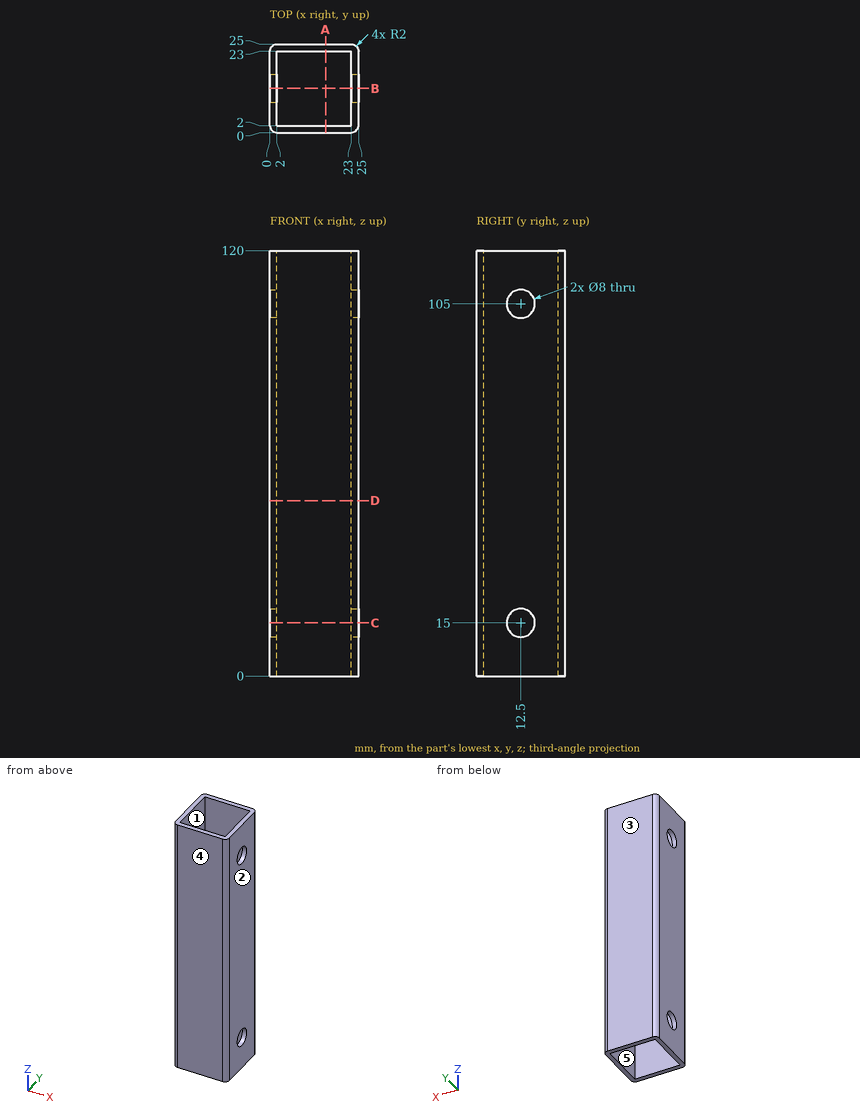
Geometry check sheet. Reference: drawing and pictorial views, mm from the part's lowest x, y, z. A direction names the side the tool comes from. Coordinates: 2 decimals unless noted, no trailing zeros. Order: outer loops, then holes, each group sorted by start corner. A loop starts at its lowest first (then second) coordinate and runs counter-clockwise, first axis right, second up.
Item 1: Section check A-A, the plane x = 15.75. Enter the section's corners in (y, z).
Filled in:
outline: (0, 0) - (2, 0) - (2, 120) - (0, 120) - close; (23, 0) - (25, 0) - (25, 120) - (23, 120) - close
Item 2: Access from +Z, -Z, +X, -X, +Y, -Y to the whole of each face (thin tool, end or side, straight path). Record for the marked faces 4 and 5.
Filled in:
face 4: +Z, -Z, +X, -X, -Y
face 5: +Z, -Z
Item 3: Material ranges on L1, parallel to X at y = 3.5, z = 106; L2, parallel to Y at x = 0.65, z = 15, recorded low to high.
Filled in:
L1: x = 0 to 2, 23 to 25
L2: y = 0.52 to 8.5, 16.5 to 24.48
Item 4: Section check C-C, the plane z = 15. Enter the section's corners in (x, y).
Filled in:
outline: (0, 2) arc R2 ccw to (2, 0) - (23, 0) arc R2 ccw to (25, 2) - (25, 8.5) - (23, 8.5) - (23, 2) - (2, 2) - (2, 8.5) - (0, 8.5) - close; (0, 16.5) - (2, 16.5) - (2, 23) - (23, 23) - (23, 16.5) - (25, 16.5) - (25, 23) arc R2 ccw to (23, 25) - (2, 25) arc R2 ccw to (0, 23) - close
Item 5: Release check for a two-part mould opening along Y. For the marked faces 1, 2 and 3 record: +Y half, -Y half, draft (parallel to the pull), parting line (faces both ways), or undercut.
Filled in:
face 1: undercut
face 2: draft
face 3: +Y half
Item 6: Section check B-B, the plane y = 12.5. Enter the section's corners in (x, z), then the cut area to 3 significant figures.
Filled in:
outline: (0, 0) - (2, 0) - (2, 11) - (0, 11) - close; (0, 19) - (2, 19) - (2, 101) - (0, 101) - close; (0, 109) - (2, 109) - (2, 120) - (0, 120) - close; (23, 0) - (25, 0) - (25, 11) - (23, 11) - close; (23, 19) - (25, 19) - (25, 101) - (23, 101) - close; (23, 109) - (25, 109) - (25, 120) - (23, 120) - close
area: 416 mm2
Item 7: Depth check by flat-ended pin: pin 1 (7 mm diameter, centred on y = 12.5, z = 15, fed in from +X). Enter the tip coordinate at first touch or a pass-through.
Filled in:
pin 1: passes through
Item 8: Section check D-D, the plane z = 49.5. Enter the section's corners in (x, y), then the cut area to 3 significant figures.
Filled in:
outline: (0, 2) arc R2 ccw to (2, 0) - (23, 0) arc R2 ccw to (25, 2) - (25, 23) arc R2 ccw to (23, 25) - (2, 25) arc R2 ccw to (0, 23) - close; hole (2, 2) - (23, 2) - (23, 23) - (2, 23) - close
area: 181 mm2
